Model file for the job. Use its own axes, mm. A direction names the side the tool comes from. Coordinates: 2 decimals unless noted, no trailing zeros. Write each loop counter-clockwise with the first axis right and the second up, starting at its lowest first coordinate (ties: lowest second). Pieces come first, ordered by that corner, then holes.
Q1. Band-saw the part on B-B, the plane x = 0. Write the cut outline in (y, z).
Q2. Band-saw the part on C-C, the plane y = -3.75. Write the cut outline in (x, z).
Q3. Band-saw the part on A-A, the plane z = 3.5. Write the cut outline in (x, y).
Q4. Pull direction Y, two halves, no side cores. Call faces 3 (the flat face through (5, -2, 8)), 4 (the flat face through (0, 8, 3)), 5 (the cylindrical face through (6.697, -6.738, 3.451)), 6 (the cylindrical face through (-1.08, -4.88, 3.94)): released by +Y, released by -Y, zero draft, split by the parting line, or undercut.
Q5. Drill centre lines: probe 1 along Y at (x, z) = (0, 3.25); probe 2 along X at (y, z) = (-3, 6.5); probe 3 along X at (y, z) = (-0.25, 1.25). Where is each one in solid material? Low to high.
Q6. Which spindle directions (+Z, -Z, +X, -X, +Y, -Y) get a long thin tool onto all of the face, cutting with end or side? Do faces 1 (the flat face through (-4, 4, 0)), 2 (the flat face through (-5, -6, 7)). Say none if no direction does.
Q7. Pin check, flat tips, straight feed: P1, Ø4, axis at x = 3.5, y = 6, coming from the -Z side; P2, Ø5, axis at x = -1, y = 0.5, coming from the +Z side. Stop position of each tip, or through.
Q8. Band-saw the part on D-D, the plane x = -6.25. Write the cut outline in (y, z).
from build123d import *

# Parameters (mm, degrees)
SKIZZE1_R                       = 9.5
SKIZZE1_R_2                     = 5
AUFSATZ_LINEAR_AUSTRAGEN1_DEPTH = 8
SKIZZE2_OUTSIDE_W               = 26.608
SKIZZE2_OUTSIDE_H               = 26.608
SKIZZE2_OUTSIDE_W_2             = 16
SKIZZE2_OUTSIDE_H_2             = 16
SCHNITT_LINEAR_AUSTRAGEN1_DEPTH = 28
SKIZZE3_OUTSIDE_W               = 22.8
SKIZZE3_OUTSIDE_H               = 22.8
SKIZZE3_OUTSIDE_R               = 7.5
SCHNITT_LINEAR_AUSTRAGEN2_DEPTH = 1


with BuildPart() as part:
    # Skizze1 → Aufsatz-Linear austragen1 (new body)
    with BuildSketch(Plane.XY):
        Circle(SKIZZE1_R)
        Circle(SKIZZE1_R_2, mode=Mode.SUBTRACT)
    extrude(amount=AUFSATZ_LINEAR_AUSTRAGEN1_DEPTH)

    # Skizze2 outside → Schnitt-Linear austragen1 (cut)
    with BuildSketch(Plane(origin=(0, 0, 0), x_dir=(-1, 0, 0), z_dir=(0, 0, -1))):
        Rectangle(SKIZZE2_OUTSIDE_W, SKIZZE2_OUTSIDE_H)
        Rectangle(SKIZZE2_OUTSIDE_W_2, SKIZZE2_OUTSIDE_H_2, mode=Mode.SUBTRACT)
    extrude(amount=-SCHNITT_LINEAR_AUSTRAGEN1_DEPTH, mode=Mode.SUBTRACT)

    # Skizze3 outside → Schnitt-Linear austragen2 (cut)
    with BuildSketch(Plane.XY.offset(8)):
        Rectangle(SKIZZE3_OUTSIDE_W, SKIZZE3_OUTSIDE_H)
        Circle(SKIZZE3_OUTSIDE_R, mode=Mode.SUBTRACT)
    extrude(amount=-SCHNITT_LINEAR_AUSTRAGEN2_DEPTH, mode=Mode.SUBTRACT)


solid = part.part
Answer sheet:
1. outline: (-8, 0) - (-5, 0) - (-5, 8) - (-7.5, 8) - (-7.5, 7) - (-8, 7) - close; (5, 0) - (8, 0) - (8, 7) - (7.5, 7) - (7.5, 8) - (5, 8) - close
2. outline: (-8, 0) - (-3.31, 0) - (-3.31, 8) - (-6.5, 8) - (-6.5, 7) - (-8, 7) - close; (3.31, 0) - (8, 0) - (8, 7) - (6.5, 7) - (6.5, 8) - (3.31, 8) - close
3. outline: (-8, -5.12) arc R9.5 ccw to (-5.12, -8) - (5.12, -8) arc R9.5 ccw to (8, -5.12) - (8, 5.12) arc R9.5 ccw to (5.12, 8) - (-5.12, 8) arc R9.5 ccw to (-8, 5.12) - close; hole circle Ø10 at (0, 0)
4. face 3: zero draft
4. face 4: released by +Y
4. face 5: released by -Y
4. face 6: undercut
5. probe 1: y = -8 to -5, 5 to 8
5. probe 2: x = -8 to -4, 4 to 8
5. probe 3: x = -8 to -4.99, 4.99 to 8
6. face 1: -Z, +X, -X, +Y, -Y
6. face 2: +Z
7. P1: stops at z = 0
7. P2: passes through
8. outline: (-7.15, 0) - (7.15, 0) - (7.15, 7) - (4.15, 7) - (4.15, 8) - (-4.15, 8) - (-4.15, 7) - (-7.15, 7) - close
